Here's the drawing with two shaded views (mm, measured from the low corner). I have some questions. A direction names the side the tool comes from. Coordinates: 2 decimals unless noted, no trailing zeros. Write each loop counter-clockwise with the first axis right and the second up, starting at its lowest first coordinate (ties: lowest second). Pieces come first, ordered by that corner, then holes.
Item 1: If we section it at C-C (z = 25): Please give me the cut outline in (x, y).
Item 2: If we section it at D-D (x = 18.5): Please give me the cut outline in (y, z), then the cut area to 3 significant figures.
Item 3: I'm going to push flat-ended pins straight in: pin 1 Ø3 at (y, z) = (25.5, 6) entering from +X; pin 2 Ø10 at (x, y) = (31.5, 17.5) entering from -Z; pin 3 Ø20 at (x, y) = (43.5, 28.5) entering from +Z. Where does each tip first touch, or does it pass through?
Item 4: For the marked faces 1 and 2, which set-ups out of +Z, -Z, +X, -X, +Y, -Y let a thin tool reach every point of the face, with its end or its side?
Item 5: If we section it at B-B (x = 37): Please give me the cut outline in (y, z), then the cut area to 3 significant figures.
Item 6: If I drill on line 1 (Y direction, x = 40, z = 2); line 2 (Z direction, x = 10, y = 20); line 3 (X direction, y = 9.5, z = 21), over which ranges is the centre line in solid material (lowest first)?
Item 7: We'd pull the mould along Y, two halves only. Please class the marked faces 3, 4, 5 and 6: +Y half, -Y half, draft (parallel to the pull), parting line (faces both ways), or undercut.
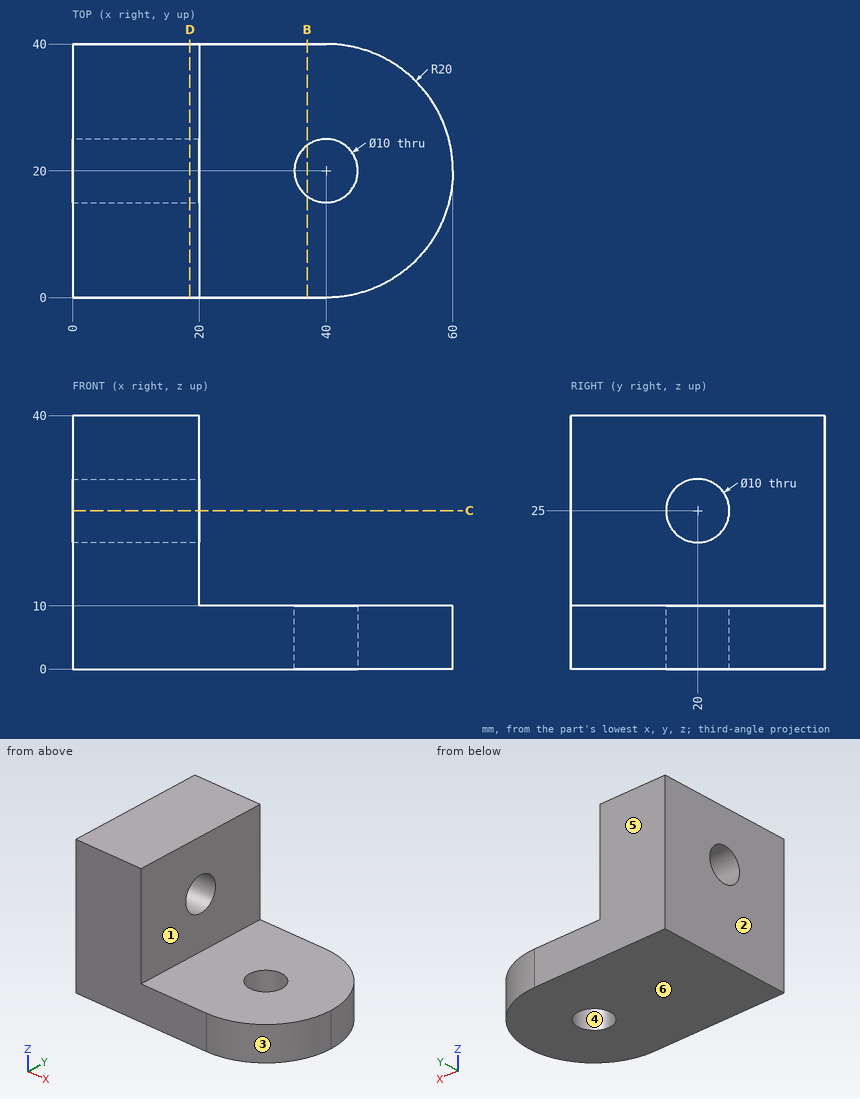
Answer list:
1. outline: (0, 0) - (20, 0) - (20, 15) - (0, 15) - close; (0, 25) - (20, 25) - (20, 40) - (0, 40) - close
2. outline: (0, 0) - (40, 0) - (40, 40) - (0, 40) - close; hole circle Ø10 at (20, 25)
2. area: 1,520 mm2
3. pin 1: stops at x = 59.6
3. pin 2: stops at z = 0
3. pin 3: stops at z = 10
4. face 1: +Z, +X, +Y, -Y
4. face 2: +Z, -Z, -X, +Y, -Y
5. outline: (0, 0) - (16, 0) - (16, 10) - (0, 10) - close; (24, 0) - (40, 0) - (40, 10) - (24, 10) - close
5. area: 320 mm2
6. line 1: y = 0 to 15, 25 to 40
6. line 2: z = 0 to 20, 30 to 40
6. line 3: x = 0 to 20
7. face 3: -Y half
7. face 4: undercut
7. face 5: +Y half
7. face 6: draft
